from build123d import *

# Parameters (mm, degrees)
BOSS_EXTRUDE2_DEPTH = 5
SKETCH3_R           = 2
CUT_EXTRUDE1_DEPTH  = 18
SKETCH6_R           = 2
SKETCH6_R_2         = 1.596148068
SKETCH6_R_3         = 1.596152716
SKETCH6_R_4         = 1.546268175
SKETCH6_R_5         = 1.546272671
BOSS_EXTRUDE3_DEPTH = 5
SKETCH9_W           = 2
SKETCH9_H           = 27
BOSS_EXTRUDE5_DEPTH = 25


with BuildPart() as part:
    # Sketch2 → Boss-Extrude2 (new body)
    with BuildSketch(Plane(origin=(0, 0, 0), x_dir=(1, 0, 0), z_dir=(0, 1, 0))):
        Polygon((-113.562992126, 63.956692913), (-113.562992126, 78.956692913), (-28.562992126, 78.956692913), (-28.562992126, -1.043307087), (-113.562992126, -1.043307087), (-113.562992126, 13.956692913), (-158.562992126, 13.956692913), (-158.562992126, 63.956692913), align=None)
    extrude(amount=BOSS_EXTRUDE2_DEPTH)

    # Sketch3 → Cut-Extrude1 (cut)
    with BuildSketch(Plane(origin=(0, 5, 0), x_dir=(1, 0, 0), z_dir=(0, 1, 0))):
        with Locations(Location((-74.562992126, 38.956692913, 0), (0, 0, 270))):
            Circle(SKETCH3_R)
        with Locations(Location((-152.562992126, 38.956692913, 0), (0, 0, 270))):
            Circle(SKETCH3_R)
    extrude(amount=-CUT_EXTRUDE1_DEPTH, mode=Mode.SUBTRACT)

    # Sketch6 → Boss-Extrude3 (add)
    # profile 1 of 4: a face of its own
    with BuildSketch(Plane(origin=(0, 5, 0), x_dir=(1, 0, 0), z_dir=(0, 1, 0))):
        with Locations(Location((-107.006745746, 63.623929763, 0), (0, 0, 270))):
            Circle(SKETCH6_R)
        with Locations(Location((-107.006745746, 63.623929763, 0), (0, 0, 270))):
            Circle(SKETCH6_R_2, mode=Mode.SUBTRACT)
    # profile 2 of 4: a face of its own
    with BuildSketch(Plane(origin=(0, 5, 0), x_dir=(1, 0, 0), z_dir=(0, 1, 0))):
        with Locations(Location((-107.006746212, 14.623929182, 0), (0, 0, 270))):
            Circle(SKETCH6_R)
        with Locations(Location((-107.006746212, 14.623929182, 0), (0, 0, 270))):
            Circle(SKETCH6_R_3, mode=Mode.SUBTRACT)
    # profile 3 of 4: a face of its own
    with BuildSketch(Plane(origin=(0, 5, 0), x_dir=(1, 0, 0), z_dir=(0, 1, 0))):
        with Locations(Location((-55.206742331, 19.873926739, 0), (0, 0, 270))):
            Circle(SKETCH6_R)
        with Locations(Location((-55.206742331, 19.873926739, 0), (0, 0, 270))):
            Circle(SKETCH6_R_4, mode=Mode.SUBTRACT)
    # profile 4 of 4: a face of its own
    with BuildSketch(Plane(origin=(0, 5, 0), x_dir=(1, 0, 0), z_dir=(0, 1, 0))):
        with Locations(Location((-55.206746033, 58.373928486, 0), (0, 0, 270))):
            Circle(SKETCH6_R)
        with Locations(Location((-55.206746033, 58.373928486, 0), (0, 0, 270))):
            Circle(SKETCH6_R_5, mode=Mode.SUBTRACT)
    extrude(amount=BOSS_EXTRUDE3_DEPTH)

    # Sketch9 → Boss-Extrude5 (add)
    with BuildSketch(Plane(origin=(0, 5, 0), x_dir=(1, 0, 0), z_dir=(0, 1, 0))):
        with Locations((-157.562992126, 38.912665697)):
            Rectangle(SKETCH9_W, SKETCH9_H)
    extrude(amount=BOSS_EXTRUDE5_DEPTH)


solid = part.part
Part model, mm, in its own coordinate system. A direction names the side the tool comes from. Coordinates: 2 decimals unless noted, no trailing zeros. Write each loop counter-clockwise with the first axis right and the second up, starting at its lowest first coordinate (ties: lowest second). Pieces come first, ordered by that corner, then holes. Notation, with made-up numbers: M -37,37 L -33,37 A15 ccw -33,60 Z; hole C 48.25,-7 d8. An arc over 180 degrees is marked long. Return JSON: item names as keys, results as strings.
1. Flat gauge pins, fed straight in: pin 1 Ø3 at (x, z) = (-55.21, -19.87) entering from +Y; pin 2 Ø10 at (x, y) = (-59, 6) entering from +Z; pin 3 Ø3 at (x, z) = (-106.5, -15.5) entering from +Y; pin 4 Ø5 at (y, z) = (18, -48.5) entering from +X. Where does each tip first touch, or does it go through?
Determined:
{"pin 1": "y = 5", "pin 2": "z = 1.04", "pin 3": "y = 10", "pin 4": "x = -156.56"}
2. Probe L1, parallel to X at y = 9, z = -58.5; L2, parallel to Y at x = -103, z = -73; L3, parallel to X at y = 25.75, z = -25.5. List the from-to ranges inside material, lowest first.
Determined:
{"L1": "-57.2 to -56.75, -53.67 to -53.21", "L2": "0 to 5", "L3": "-158.56 to -156.56"}
3. Pull direction Z, two halves, no side cores. Call faces 1 (the face through (-53.903, 7.465, -19.043)), 2 (the face through (-136, 2, -63.957)), 3 (the face through (-150.58, 2.54, -39.22)), 4 (the face through (-113.563, 2, -71)): pulls with the +Z half, pulls with the -Z half, needs draft (parallel to the pull), parting line crosses it, or undercut.
Determined:
{"face 1": "undercut", "face 2": "pulls with the -Z half", "face 3": "undercut", "face 4": "needs draft"}
4. Saw through at D-D, the plane z = -20. Write the cut outline in (x, y).
Determined:
{"outline": "M -158.56,0 L -28.56,0 L -28.56,5 L -53.21,5 L -53.21,10 L -53.67,10 L -53.67,5 L -56.75,5 L -56.75,10 L -57.2,10 L -57.2,5 L -158.56,5 Z"}
5. 3-axis set-ups, long thin cutter, end or side, ignore diameter. For faces 5 (the face through (-57, 10, -20)), 6 (the face through (-53.52, 7.46, -18.8)), 7 (the face through (-113.563, 2, -6)), 8 (the face through (-72, 2, -78.957)), 9 (the face through (-156.563, 17, -39)): which of +Z, -Z, +X, -X, +Y, -Y reach the whole face in a straight line?
Determined:
{"face 5": "+Z, -Z, +X, -X, +Y", "face 6": "+Y", "face 7": "+Z, -X, +Y, -Y", "face 8": "-Z, +X, -X, +Y, -Y", "face 9": "+Z, -Z, +X, +Y"}
6. Saw through at A-A, the plane z = -45. Write the cut outline in (x, y).
Determined:
{"outline": "M -158.56,0 L -28.56,0 L -28.56,5 L -156.56,5 L -156.56,30 L -158.56,30 Z"}
7. Saw through at B-B, the plane y = 14.75. Write the cut outline in (x, z).
Determined:
{"outline": "M -158.56,-52.41 L -156.56,-52.41 L -156.56,-25.41 L -158.56,-25.41 Z"}
8. Saw through at C-C, the plane x = -126.5. Write the cut outline in (y, z).
Determined:
{"outline": "M 0,-63.96 L 5,-63.96 L 5,-13.96 L 0,-13.96 Z"}
